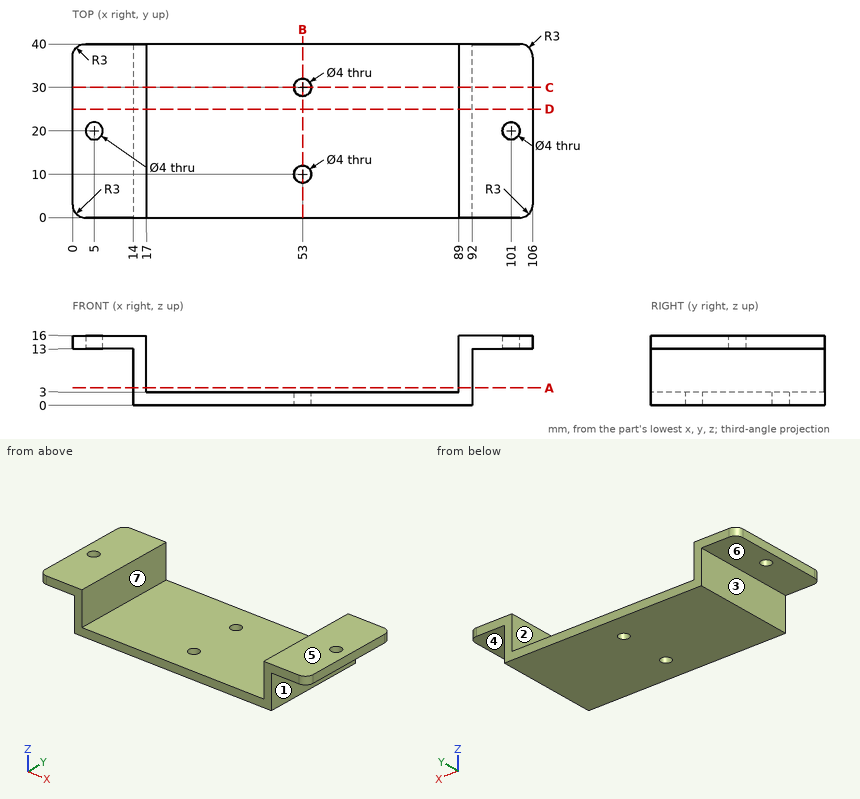
Geometry: see drawing. Coordinates: mm, zero at the bounding-box minimum. A direction names the side the tool comes from. Give positions to 0.01 mm unless a question says otherwise; leave off trailing zeros. Loops run counter-clockwise (first coordinate to the right, second up) from the corner with the lowest first, then second, coordinate; pieces in that order, holes last. Notation, with made-up numbers: (79, -1) - (124, -1) arc R23 ccw to (124, 13) - close; hole circle Ø7 at (-40, 65). An arc over 180 degrees is marked (long way). Answer as CSV lines item,"result". Start each with the question number.
1. Section D-D, the plane y = 25. Return loops of the section in (x, z).
2. Ray query, L1, parallel to Y at x = 53, z = 1.75; L2, parallel to X at y = 20, z = 14.2; L3, parallel to Y at x = 101, z = 13.9. Return the intervals inside material, ascending.
3. Pin query (flat end, axial travel): P1, Ø12, axis at x = 66, y = 19.5, coming from the +Z side; P2, Ø6, axis at x = 68.5, z = 7.5, coming from the -Y side; P3, Ø7, axis at x = 7.5, y = 16, coming from the -Z side; P4, Ø4, axis at y = 30, z = 9.5, coming from the -X side. Return the tip coordinate at first contact, or that it passes through.
4. Reachability of the marked faces 4, 5, 6 and 7 from +Z, -Z, +X, -X, +Y, -Y: full face, straight path, thin tool, end or side. Return the list, or none.
5. Section A-A, the plane z = 4. Return loops of the section in (x, y), plus the area to 3 significant figures.
6. Draft query along X for the marked faces 1, 2 and 3. Return one class per face: released by +X, released by -X, zero draft, split by the parting line, or undercut.
7. Section C-C, the plane y = 30. Return loops of the section in (x, z).
8. Section B-B, the plane x = 53. Return loops of the section in (y, z), plus the area to 3 significant figures.
Answers:
1,outline,"(0, 13) - (14, 13) - (14, 0) - (92, 0) - (92, 13) - (106, 13) - (106, 16) - (89, 16) - (89, 3) - (17, 3) - (17, 16) - (0, 16) - close"
2,L1,"y = 0 to 8, 12 to 28, 32 to 40"
2,L2,"x = 0 to 3, 7 to 17, 89 to 99, 103 to 106"
2,L3,"y = 0 to 18, 22 to 40"
3,P1,"stops at z = 3"
3,P2,"passes through"
3,P3,"stops at z = 13"
3,P4,"stops at x = 14"
4,face 4,"-Z, +X, +Y, -Y"
4,face 5,"+Z, +X, -X, +Y, -Y"
4,face 6,"-Z, -X, +Y, -Y"
4,face 7,"+Z, +Y, -Y"
5,outline,"(14, 0) - (17, 0) - (17, 40) - (14, 40) - close; (89, 0) - (92, 0) - (92, 40) - (89, 40) - close"
5,area,"240 mm2"
6,face 1,"released by +X"
6,face 2,"undercut"
6,face 3,"released by -X"
7,outline,"(0, 13) - (14, 13) - (14, 0) - (51, 0) - (51, 3) - (17, 3) - (17, 16) - (0, 16) - close; (55, 0) - (92, 0) - (92, 13) - (106, 13) - (106, 16) - (89, 16) - (89, 3) - (55, 3) - close"
8,outline,"(0, 0) - (8, 0) - (8, 3) - (0, 3) - close; (12, 0) - (28, 0) - (28, 3) - (12, 3) - close; (32, 0) - (40, 0) - (40, 3) - (32, 3) - close"
8,area,"96.0 mm2"
